from build123d import *

# Parameters (mm, degrees)
BASE_FLANGE1_DEPTH            = 118
M3_CLEARANCE_HOLE1_AT_2_COUNT = 2
M3_CLEARANCE_HOLE1_AT_2_PITCH = 15
M3_CLEARANCE_HOLE2_AT_2_COUNT = 2
M3_CLEARANCE_HOLE2_AT_2_PITCH = 16
M3_CLEARANCE_HOLE2_AT_3_COUNT = 2
M3_CLEARANCE_HOLE2_AT_3_PITCH = 32


# Sheet-metal steps are written as plain solids
with BuildPart() as part:
    # Sketch1 → Base-Flange1 (new, symmetric)
    with BuildSketch(Plane(origin=(0, 0, 0), x_dir=(1, 0, 0), z_dir=(0, 1, 0))):
        with BuildLine():
            Line((0, -10), (0, -2.2366))
            ThreePointArc((0, -2.2366), (0.655084973, -0.655084973), (2.2366, 0))
            Line((2.2366, 0), (10, 0))
            Line((10, 0), (10, -1.5))
            Line((10, -1.5), (2.2366, -1.5))
            ThreePointArc((2.2366, -1.5), (1.715745145, -1.715745145), (1.5, -2.2366))
            Line((1.5, -2.2366), (1.5, -10))
            Line((1.5, -10), (0, -10))
        make_face()
    extrude(amount=BASE_FLANGE1_DEPTH, both=True)

    # Sketch9 → M3 Clearance Hole1 (revolve, cut)
    with BuildSketch(Plane(origin=(6.1183, 113, 1.5), x_dir=(0, -1, 0), z_dir=(1, 0, 0))):
        Polygon((0, 0), (0, 1.5), (1.7, 1.5), (1.7, 0.125), (1.825, 0), align=None)
    m3_clearance_hole1 = revolve(axis=Axis((6.1183, 113, 7.85), (0, 0, -1)), mode=Mode.SUBTRACT)

    # M3 Clearance Hole1 at 2: M3 Clearance Hole1 ×2
    with Locations(*[(0, -i * M3_CLEARANCE_HOLE1_AT_2_PITCH, 0) for i in range(1, M3_CLEARANCE_HOLE1_AT_2_COUNT)]):
        add(m3_clearance_hole1, mode=Mode.SUBTRACT)

    # Sketch12 → M3 Clearance Hole2 (revolve, cut)
    with BuildSketch(Plane(origin=(1.5, -115, 5), x_dir=(0, 0, -1), z_dir=(0, 1, 0))):
        Polygon((0, 0), (0, 1.5), (1.7, 1.5), (1.7, 0.125), (1.825, 0), align=None)
    m3_clearance_hole2 = revolve(axis=Axis((7.85, -115, 5), (-1, 0, 0)), mode=Mode.SUBTRACT)

    # M3 Clearance Hole2 at 2: M3 Clearance Hole2 ×2
    with Locations(*[(0, i * M3_CLEARANCE_HOLE2_AT_2_PITCH, 0) for i in range(1, M3_CLEARANCE_HOLE2_AT_2_COUNT)]):
        add(m3_clearance_hole2, mode=Mode.SUBTRACT)

    # M3 Clearance Hole2 at 3: M3 Clearance Hole2 ×2
    with Locations(*[(0, i * M3_CLEARANCE_HOLE2_AT_3_PITCH, 0) for i in range(1, M3_CLEARANCE_HOLE2_AT_3_COUNT)]):
        add(m3_clearance_hole2, mode=Mode.SUBTRACT)


solid = part.part
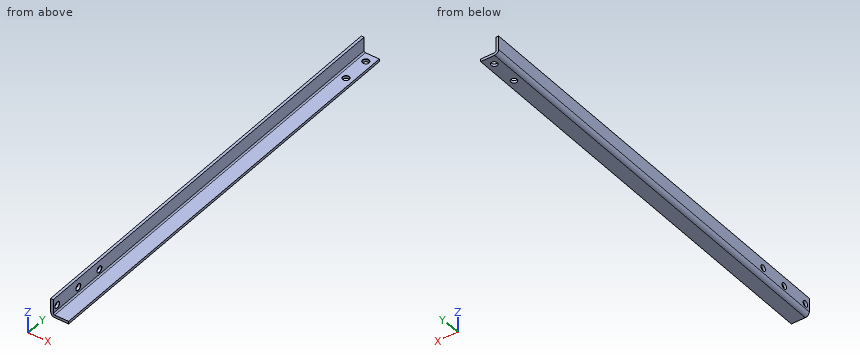
Geometry: final body of the model. Coordinates: model frame, mm. Give positions to 0.01 mm unless a question says otherwise; leave off trailing zeros. Write each loop counter-clockwise with the first axis right and the second up, starting at its lowest first coordinate (ties: lowest second). Pieces come first, ordered by that corner, then holes. Notation, with made-up numbers: (-8, 41.25) - (29, 41.25) arc R28 cw to (29, 71.25) - close; hole circle Ø11 at (-7, -8.5). An arc over 180 degrees is marked (long way). Return JSON: item names as keys, results as strings. Group by question number.
1) First-contact query: P1, Ø1, axis at x = 4.5, y = -66, coming from the +Z side; P2, Ø4, axis at y = -115, z = 5, coming from the +X side. Flat tips, straight axial feed; report the tip coordinate or a pass-through.
2) Section A-A on y = -57. Return the cut outline in (x, z).
3) Line query: line 1 (Y direction, x = 7.5, z = 1.25); line 2 (Z direction, x = 6.75, y = -1). Output: solid intervals per line, ascending.
4) Section B-B on z = 8.5. Return the cut outline in (x, y).
Filled in:
{
 "1": {"P1": "stops at z = 1.5", "P2": "stops at x = 1.5"},
 "2": {"outline": "(0, 2.24) arc R2.24 ccw to (2.24, 0) - (10, 0) - (10, 1.5) - (2.24, 1.5) arc R0.74 cw to (1.5, 2.24) - (1.5, 10) - (0, 10) - close"},
 "3": {"line 1": "y = -118 to 97.01, 98.99 to 112.01, 113.99 to 118", "line 2": "z = 0 to 1.5"},
 "4": {"outline": "(0, -118) - (1.5, -118) - (1.5, 118) - (0, 118) - close"}
}
